```python
from build123d import *

# Parameters (mm, degrees)
SKETCH2_R               = 10
BOSS_EXTRUDE1_DEPTH     = 45
CUT_EXTRUDE2_DEPTH      = 147.050606819
CUT_EXTRUDE2_DEPTH_BACK = 147.050606819
CHAMFER1_SIZE           = 5


with BuildPart() as part:
    # Sketch2 → Boss-Extrude1 (new body)
    with BuildSketch(Plane.XY):
        with BuildLine():
            ThreePointArc((-25.980762114, -15), (0, -30), (25.980762114, -15))
            Line((25.980762114, -15), (59.329684168, 42.762027375))
            ThreePointArc((59.329684168, 42.762027375), (60.583878744, 49.067289298), (57.740497942, 54.833095187))
            Line((57.740497942, 54.833095187), (33.786796564, 78.786796564))
            ThreePointArc((33.786796564, 78.786796564), (27.283614025, 88.519497029), (25, 100))
            ThreePointArc((25, 100), (18.955379316, 116.300110275), (3.744512401, 124.717981853))
            ThreePointArc((3.744512401, 124.717981853), (0, 125), (-3.744512401, 124.717981853))
            ThreePointArc((-3.744512401, 124.717981853), (-18.955379316, 116.300110275), (-25, 100))
            ThreePointArc((-25, 100), (-27.283614025, 88.519497029), (-33.786796564, 78.786796564))
            Line((-33.786796564, 78.786796564), (-57.740497942, 54.833095187))
            ThreePointArc((-57.740497942, 54.833095187), (-60.583878744, 49.067289298), (-59.329684168, 42.762027375))
            Line((-59.329684168, 42.762027375), (-25.980762114, -15))
        make_face()
        with Locations(Location((0, 0, 0), (0, 0, 180))):
            Circle(SKETCH2_R, mode=Mode.SUBTRACT)
        with Locations(Location((0, 100, 0), (0, 0, 180))):
            Circle(SKETCH2_R, mode=Mode.SUBTRACT)
    extrude(amount=BOSS_EXTRUDE1_DEPTH)

    # Sketch3 → Cut-Extrude2 (cut, two sides: drawn at the far end of the back side and taken through both)
    with BuildSketch(Plane(origin=(0, 0, 0), x_dir=(0, 0, -1), z_dir=(1, 0, 0)).offset(-CUT_EXTRUDE2_DEPTH_BACK)):
        with BuildLine():
            Line((-12, 125), (-12, 81.354156504))
            ThreePointArc((-12, 81.354156504), (-8.794494718, 69.10670779), (0, 60))
            Line((0, 60), (0, 125))
            Line((0, 125), (-12, 125))
        make_face()
        with BuildLine():
            Line((-35, -30), (-22.5, -30))
            Line((-22.5, -30), (-22.5, 62))
            Line((-22.5, 62), (-29.704718934, 62))
            ThreePointArc((-29.704718934, 62), (-33.449048084, 60.449048084), (-35, 56.704718934))
            Line((-35, 56.704718934), (-35, -30))
        make_face()
        with BuildLine():
            Line((-22.5, -30), (-10, -30))
            Line((-10, -30), (-10, 56.704718934))
            ThreePointArc((-10, 56.704718934), (-11.550951916, 60.449048084), (-15.295281066, 62))
            Line((-15.295281066, 62), (-22.5, 62))
            Line((-22.5, 62), (-22.5, -30))
        make_face()
        with BuildLine():
            Line((-33, 125), (-33, 81.354156504))
            ThreePointArc((-33, 81.354156504), (-36.205505282, 69.10670779), (-45, 60))
            Line((-45, 60), (-45, 125))
            Line((-45, 125), (-33, 125))
        make_face()
    extrude(amount=CUT_EXTRUDE2_DEPTH + CUT_EXTRUDE2_DEPTH_BACK, mode=Mode.SUBTRACT)

    # Chamfer1
    chamfer1_edges = [part.edges().sort_by_distance(p)[0] for p in [
        (10, 100, 12),
        (10, 0, 0),
        (10, 0, 45),
        (10, 100, 33),
    ]]
    chamfer(chamfer1_edges, length=CHAMFER1_SIZE)


solid = part.part
```
For this review, take the finished solid that the model builds, in its own axes (mm). A direction names the side the tool comes from. Round coordinates to 2 decimals unless told otherwise and drop trailing zeros. Write each loop counter-clockwise with the first axis right and the second up, starting at its lowest first coordinate (ties: lowest second). Pieces come first, ordered by that corner, then holes.
1) Mouldability with a two-part tool opening along X and no side actions: class faces 1 (the face through (1.302, 90.085, 22.423)), 2 (the face through (-42.89, 14.29, 4.93)), 3 (the face through (-0.7, 69.3, 36.1)) as +X half, -X half, draft (parallel to the pull), parting line (faces both ways), or undercut.
Answer below:
face 1: undercut
face 2: -X half
face 3: draft
2) Take a section at B-B on y = 0. Give the boundary of the cut face in (x, z).
Answer below:
outline: (-34.64, 0) - (-15, 0) - (-10, 5) - (-10, 10) - (-34.64, 10) - close; (-34.64, 35) - (-10, 35) - (-10, 40) - (-15, 45) - (-34.64, 45) - close; (10, 5) - (15, 0) - (34.64, 0) - (34.64, 10) - (10, 10) - close; (10, 35) - (34.64, 35) - (34.64, 45) - (15, 45) - (10, 40) - close
3) Take a section at C-C on z = 22. Give the boundary of the cut face in (x, y).
Answer below:
outline: (-50.57, 62) - (50.57, 62) - (33.79, 78.79) arc R30 cw to (25, 100) arc R25 ccw to (-25, 100) arc R30 cw to (-33.79, 78.79) - close; hole circle Ø20 at (0, 100)
4) Take a section at D-D on x = 17.5. Give the boundary of the cut face in (y, z).
Answer below:
outline: (-24.37, 0) - (60, 0) arc R25 cw to (81.35, 12) - (117.85, 12) - (117.85, 33) - (81.35, 33) arc R25 cw to (60, 45) - (-24.37, 45) - (-24.37, 35) - (56.7, 35) arc R5.3 cw to (62, 29.7) - (62, 15.3) arc R5.3 cw to (56.7, 10) - (-24.37, 10) - close
5) For line 1 along Z through (x, y) = (26, 39.5); line 2 along Y through (x, z) = (0, 21.25); line 3 along Y through (x, z) = (0, 37), list the stretches that pass through material, from the lowest coordinate up.
Answer below:
line 1: z = 0 to 10, 35 to 45
line 2: y = 62 to 90, 110 to 125
line 3: y = -30 to -10, 10 to 67.79
6) Insertion check: pin 1 Ø8 at (x, z) = (7.5, 21) entering from -Y; pin 2 Ø4 at (y, z) = (27.5, 5) entering from +X; pin 3 Ø6 at (x, z) = (-22, 23.5) entering from +Y; pin 4 Ø2 at (x, y) = (-34, 20) entering from -Z. Each pin has a flat end and moves straight along its axis. Give the tip position at first contact, or say it passes through.
Answer below:
pin 1: stops at y = 62
pin 2: stops at x = 51.67
pin 3: stops at y = 116.25
pin 4: stops at z = 0
7) Take a section at A-A on x = 0. State how many separate pieces and enclosed holes the cut face has, then the cut area to 3 significant figures.
Answer below:
separate pieces: 4
enclosed holes: 0
area: 2,360 mm2
8) Machinability: for faces 4 (the face through (14, 108, 12)), 5 (the face through (-45.596, 66.978, 22.185)), 6 (the face through (-1, 22, 10)), 7 (the face through (14, 108, 33)), which of the approach directions +Z, -Z, +X, -X, +Y, -Y give a long, thin tool a straight path to every point of the face, cutting with its end or side? Answer none if there is none.
Answer below:
face 4: -Z, +X, -X, +Y
face 5: +Z, -Z, -X, +Y
face 6: +X, -X, -Y
face 7: +Z, +X, -X, +Y
